Model file for the job. Use its own axes, mm. Face numbers are marked on the shaded views. A direction names the side the tool comes from. Coordinates: 2 decimals unless noted, no trailing zeros. Order: outer loops, then holes, each group sorted by start corner. A loop starts at its lowest first (then second) coordinate and runs counter-clockwise, first axis right, second up.
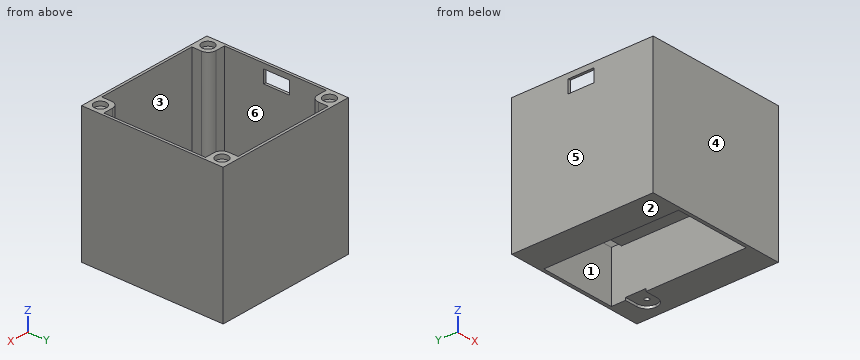
from build123d import *

# Parameters (mm, degrees)
SKICA1_W                  = 55.6
SKICA1_H                  = 55.6
P_IDAT_VYSUNUT_M2_DEPTH   = 3
SKICA14_W                 = 53.6
SKICA14_H                 = 1
P_IDAT_VYSUNUT_M9_DEPTH   = 50
SKICA19_W                 = 7.8
SKICA19_H                 = 7.8
P_IDAT_VYSUNUT_M10_DEPTH  = 53
SKICA20_R                 = 2.4
ODEBRAT_VYSUNUT_M9_DEPTH  = 1.7
ZAOBLIT1_R                = 3
SKICA25_W                 = 32
SKICA25_H                 = 55.6
P_IDAT_VYSUNUT_M12_DEPTH  = 20
SKICA26_W                 = 30
SKICA26_H                 = 53
ODEBRAT_VYSUNUT_M11_DEPTH = 19
SKICA27_W                 = 5.08
SKICA27_H                 = 10.16
ODEBRAT_VYSUNUT_M12_DEPTH = 1
SKICA28_W                 = 9
SKICA28_H                 = 8
ODEBRAT_VYSUNUT_M13_DEPTH = 1
ZAOBLIT3_R                = 4
SKICA29_W                 = 0.5
SKICA29_H                 = 4
ODEBRAT_VYSUNUT_M14_DEPTH = 2
SKICA30_R                 = 0.9
ODEBRAT_VYSUNUT_M15_DEPTH = 2
SKICA31_W                 = 6
SKICA31_H                 = 4
ODEBRAT_VYSUNUT_M16_DEPTH = 2
ZAOBLIT4_R                = 1


with BuildPart() as part:
    # Skica1 → Přidat vysunutím2 (new body)
    with BuildSketch(Plane.XY):
        Rectangle(SKICA1_W, SKICA1_H)
    extrude(amount=P_IDAT_VYSUNUT_M2_DEPTH)

    # Skica14 → Přidat vysunutím9 (add)
    with BuildSketch(Plane.XY.offset(3)):
        Polygon((27.8, 27.8), (-27.8, 27.8), (-27.8, -27.8), (-26.8, -27.8), (-26.8, -26.8), (-26.8, 26.8), (26.8, 26.8), (26.8, -26.8), (26.8, -27.8), (27.8, -27.8), align=None)
        with Locations((0, -27.3)):
            Rectangle(SKICA14_W, SKICA14_H)
    extrude(amount=P_IDAT_VYSUNUT_M9_DEPTH)

    # Skica19 → Přidat vysunutím10 (add)
    with BuildSketch(Plane(origin=(0, 0, 0), x_dir=(-1, 0, 0), z_dir=(0, 0, -1))):
        with Locations((-23.9, 23.9)):
            Rectangle(SKICA19_W, SKICA19_H)
        with Locations((23.9, 23.9)):
            Rectangle(SKICA19_W, SKICA19_H)
        with Locations((-23.9, -23.9)):
            Rectangle(SKICA19_W, SKICA19_H)
        with Locations((23.9, -23.9)):
            Rectangle(SKICA19_W, SKICA19_H)
    extrude(amount=-P_IDAT_VYSUNUT_M10_DEPTH)

    # Skica20 → Odebrat vysunutím9 (cut)
    with BuildSketch(Plane.XY.offset(53)):
        with Locations((-23.9, -23.9)):
            Circle(SKICA20_R)
        with Locations((-23.9, 23.9)):
            Circle(SKICA20_R)
        with Locations((23.900280565, 23.9)):
            Circle(SKICA20_R)
        with Locations((23.900280565, -23.9)):
            Circle(SKICA20_R)
    extrude(amount=-ODEBRAT_VYSUNUT_M9_DEPTH, mode=Mode.SUBTRACT)

    # Zaoblit1
    zaoblit1_edges = [part.edges().sort_by_distance(p)[0] for p in [
        (-20, -20, 28),
        (20, 20, 28),
        (-20, 20, 28),
        (20, -20, 28),
    ]]
    fillet(zaoblit1_edges, radius=ZAOBLIT1_R)

    # Skica25 → Přidat vysunutím12 (add)
    with BuildSketch(Plane(origin=(0, 0, 0), x_dir=(-1, 0, 0), z_dir=(0, 0, -1))):
        Rectangle(SKICA25_W, SKICA25_H)
    extrude(amount=-P_IDAT_VYSUNUT_M12_DEPTH)

    # Skica26 → Odebrat vysunutím11 (cut)
    with BuildSketch(Plane(origin=(0, 0, 0), x_dir=(-1, 0, 0), z_dir=(0, 0, -1))):
        Rectangle(SKICA26_W, SKICA26_H)
    extrude(amount=-ODEBRAT_VYSUNUT_M11_DEPTH, mode=Mode.SUBTRACT)

    # Skica27 → Odebrat vysunutím12 (cut)
    with BuildSketch(Plane.ZY.offset(27.8)):
        with Locations((48.46, 0.5)):
            Rectangle(SKICA27_W, SKICA27_H)
    extrude(amount=-ODEBRAT_VYSUNUT_M12_DEPTH, mode=Mode.SUBTRACT)

    # Skica28 → Odebrat vysunutím13 (cut)
    with BuildSketch(Plane(origin=(0, 0, 0), x_dir=(-1, 0, 0), z_dir=(0, 0, -1))):
        with Locations((-19.5, 16.940262317)):
            Rectangle(SKICA28_W, SKICA28_H)
    extrude(amount=-ODEBRAT_VYSUNUT_M13_DEPTH, mode=Mode.SUBTRACT)

    # Zaoblit3
    zaoblit3_edges = [part.edges().sort_by_distance(p)[0] for p in [
        (24, 12.940262317, 0.5),
        (24, 20.940262317, 0.5),
    ]]
    fillet(zaoblit3_edges, radius=ZAOBLIT3_R - 0.0001)  # a hair under: the kernel refuses the full size

    # Skica29 → Odebrat vysunutím14 (cut)
    with BuildSketch(Plane(origin=(-15, 0, 0), x_dir=(0, 0, -1), z_dir=(1, 0, 0))):
        with Locations((-0.75, 19.5)):
            Rectangle(SKICA29_W, SKICA29_H)
        with Locations((-0.83, -19.5)):
            Rectangle(SKICA29_W, SKICA29_H)
    extrude(amount=-ODEBRAT_VYSUNUT_M14_DEPTH, mode=Mode.SUBTRACT)

    # Skica30 → Odebrat vysunutím15 (cut)
    with BuildSketch(Plane(origin=(0, 0, 1), x_dir=(-1, 0, 0), z_dir=(0, 0, -1))):
        with Locations((-20, 16.940262317)):
            Circle(SKICA30_R)
    extrude(amount=-ODEBRAT_VYSUNUT_M15_DEPTH, mode=Mode.SUBTRACT)

    # Skica31 → Odebrat vysunutím16 (cut)
    with BuildSketch(Plane(origin=(0, 0, 19), x_dir=(-1, 0, 0), z_dir=(0, 0, -1))):
        with Locations((-12, 24.5)):
            Rectangle(SKICA31_W, SKICA31_H)
    extrude(amount=-ODEBRAT_VYSUNUT_M16_DEPTH, mode=Mode.SUBTRACT)

    # Zaoblit4
    zaoblit4_edges = [part.edges().sort_by_distance(p)[0] for p in [
        (9, 22.5, 19.5),
    ]]
    fillet(zaoblit4_edges, radius=ZAOBLIT4_R)


solid = part.part
Q1. Cut at B-B, the plane z = 15. List the corners of the cut face in (x, y), plus the area to 3 significant figures.
Established:
outline: (-27.8, -27.8) - (27.8, -27.8) - (27.8, 27.8) - (-27.8, 27.8) - close; hole (-26.8, -20) - (-23, -20) arc R3 cw to (-20, -23) - (-20, -26.8) - (-16, -26.8) - (-16, 26.8) - (-20, 26.8) - (-20, 23) arc R3 cw to (-23, 20) - (-26.8, 20) - close; hole (-15, -26.5) - (15, -26.5) - (15, 26.5) - (-15, 26.5) - close; hole (16, -26.8) - (20, -26.8) - (20, -23) arc R3 cw to (23, -20) - (26.8, -20) - (26.8, 20) - (23, 20) arc R3 cw to (20, 23) - (20, 26.8) - (16, 26.8) - close
area: 521 mm2
Q2. Cut at C-C, the plane y = -23.9. List the corners of the cut face in (x, z).
Established:
outline: (-27.8, 0) - (-15, 0) - (-15, 19) - (15, 19) - (15, 0) - (27.8, 0) - (27.8, 53) - (26.3, 53) - (26.3, 51.3) - (21.5, 51.3) - (21.5, 53) - (20, 53) - (20, 3) - (16, 3) - (16, 20) - (-16, 20) - (-16, 3) - (-20, 3) - (-20, 53) - (-21.5, 53) - (-21.5, 51.3) - (-26.3, 51.3) - (-26.3, 53) - (-27.8, 53) - close
Q3. Cut at D-D, the plane z = 39.5. List the corners of the cut face in (x, y), plus the area to 3 significant figures.
Established:
outline: (-27.8, -27.8) - (27.8, -27.8) - (27.8, 27.8) - (-27.8, 27.8) - close; hole (-26.8, -20) - (-23, -20) arc R3 cw to (-20, -23) - (-20, -26.8) - (20, -26.8) - (20, -23) arc R3 cw to (23, -20) - (26.8, -20) - (26.8, 20) - (23, 20) arc R3 cw to (20, 23) - (20, 26.8) - (-20, 26.8) - (-20, 23) arc R3 cw to (-23, 20) - (-26.8, 20) - close
area: 396 mm2
Q4. Mould opens along Y. For the marked faces 4, 5 and 6 say: pulls with the +Y half, pulls with the -Y half, needs draft (parallel to the pull), parting line crosses it, or undercut.
Established:
face 4: pulls with the -Y half
face 5: needs draft
face 6: undercut
Q5. Probe line 1 (Y direction, x = -23.9, z = 52.4); line 2 (X direction, y = 4, z = 12.5); line 3 (Z direction, x = -15.5, y = 20). List the from-to ranges inside material, lowest first.
Established:
line 1: y = -27.8 to -26.3, -21.5 to -20, 20 to 21.5, 26.3 to 27.8
line 2: x = -27.8 to -26.8, -16 to -15, 15 to 16, 26.8 to 27.8
line 3: z = 0 to 0.5, 1 to 20
Q6. Cut at A-A, the plane y = 2.5. List the corners of the cut face in (x, z), plus the area to 3 significant figures.
Established:
outline: (-27.8, 0) - (-15, 0) - (-15, 19) - (15, 19) - (15, 0) - (27.8, 0) - (27.8, 53) - (26.8, 53) - (26.8, 3) - (16, 3) - (16, 20) - (-16, 20) - (-16, 3) - (-26.8, 3) - (-26.8, 45.92) - (-27.8, 45.92) - close; (-27.8, 51) - (-26.8, 51) - (-26.8, 53) - (-27.8, 53) - close
area: 236 mm2
Q7. Drop flat-ended pins along their axis: P1, Ø1, axis at x = 21, y = -20, coming from the +Z side; P2, Ø3, axis at x = -14, y = -0.5, coming from the +Z side; P3, Ø4.5, axis at x = -23.9, y = 23.9, coming from the +Z side. Give the stop position or say it passes through.
Established:
P1: stops at z = 3
P2: stops at z = 20
P3: stops at z = 51.3
Q8. Which spindle directions (+Z, -Z, +X, -X, +Y, -Y) get a long thin tool onto all of the face, cutting with end or side? Do the marked faces 1, 2 and 3. Say none if no direction does.
Established:
face 1: -Z
face 2: -Z, +X, -X, +Y, -Y
face 3: +Z
